from build123d import *

# Parameters (mm, degrees)
F0_R          = 10
F1_DEPTH      = 60
F1_DEPTH_BACK = 60
F2_R          = 2
F3_DEPTH      = 25
F5_START      = -10
F4_R          = 6
F5_DEPTH      = 15


with BuildPart() as f1:
    # F0 (on Top) → F1 (new body, two sides)
    with BuildSketch(Plane.XY) as f1_sk:
        with BuildLine():
            Line((-60, 10), (-60, 0))
            Line((-60, 0), (0, 0))
            Line((0, 0), (60, 0))
            Line((60, 0), (60, 10))
            Line((60, 10), (36.1375661614, 15.867864057))
            ThreePointArc((36.1375661614, 15.867864057), (25.2854930612, 21.0118409528), (17.3205080757, 30))
            ThreePointArc((17.3205080757, 30), (10, 37.3205080757), (0, 40))
            ThreePointArc((0, 40), (-10, 37.3205080757), (-17.3205080757, 30))
            ThreePointArc((-17.3205080757, 30), (-25.2854930612, 21.0118409528), (-36.1375661614, 15.867864057))
            Line((-36.1375661614, 15.867864057), (-60, 10))
        make_face()
        with Locations((0, 20)):
            Circle(F0_R, mode=Mode.SUBTRACT)
    extrude(amount=F1_DEPTH)
    extrude(f1_sk.sketch, amount=-F1_DEPTH_BACK)

    # F2 (on face) → F3 (cut)
    with BuildSketch(Plane.XZ):
        with Locations((-50, 50)):
            Circle(F2_R)
        with Locations((50, 50)):
            Circle(F2_R)
        with Locations((-50, -50)):
            Circle(F2_R)
        with Locations((50, -50)):
            Circle(F2_R)
    extrude(amount=-F3_DEPTH, mode=Mode.SUBTRACT)

    # F4 (on face) → F5 (cut)
    with BuildSketch(Plane.XZ.offset(F5_START)):
        with Locations((-50, 50)):
            Circle(F4_R)
        with Locations((50, -50)):
            Circle(F4_R)
        with Locations((-50, -50)):
            Circle(F4_R)
        with Locations((50, 50)):
            Circle(F4_R)
    extrude(amount=-F5_DEPTH, mode=Mode.SUBTRACT)


solid = f1.part
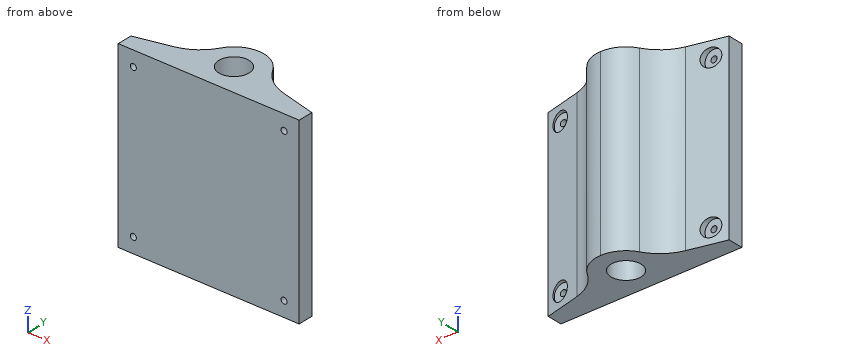
Geometry check sheet. Reference: the model listing, model coordinates, mm. Give positions to 0.01 mm unless a question says otherwise; leave off trailing zeros. Loops run counter-clockwise (first coordinate to the right, second up) from the corner with the lowest first, then second, coordinate; pieces in that order, holes last.
(1) Thickness scan on L1, parallel to Z at x = -50, y = 5.5; L2, parallel to Z at x = 45.5, y = 13.5; L3, parallel to X at y = 11.4, z = 50. Record the ranges inside material, lowest first.
From the geometry:
L1: z = -60 to -52, -48 to 48, 52 to 60
L2: z = -60 to -53.97, -46.03 to 46.03, 53.97 to 60
L3: x = -44 to -5.1, 5.1 to 44
(2) Section check A-A on z = 10. Record the cut outline in (x, y), then the cut area to 3 significant figures.
From the geometry:
outline: (-60, 0) - (60, 0) - (60, 10) - (36.14, 15.87) arc R30 cw to (17.32, 30) arc R20 ccw to (-17.32, 30) arc R30 cw to (-36.14, 15.87) - (-60, 10) - close; hole circle Ø20 at (0, 20)
area: 2,380 mm2
(3) Section check C-C on x = 6. Record the cut outline in (y, z), then the cut area to 3 significant figures.
From the geometry:
outline: (0, -60) - (12, -60) - (12, 60) - (0, 60) - close; (28, -60) - (39.08, -60) - (39.08, 60) - (28, 60) - close
area: 2,770 mm2
(4) Depth check by flat-ended pin: pin 1 Ø1.5 at (y, z) = (22, -0.5) entering from -X; pin 2 Ø8 at (x, z) = (-46, -26) entering from +Y; pin 3 Ø3.5 at (x, z) = (47.5, 49) entering from +Y; pin 4 Ø3 at (x, z) = (-50, 50) entering from -Y. Enter the tip coordinate at first touch or a pass-through.
From the geometry:
pin 1: stops at x = -24.97
pin 2: stops at y = 14.43
pin 3: stops at y = 10
pin 4: passes through
(5) Section check D-D on y = 20. Record the cut outline in (x, z).
From the geometry:
outline: (-26.72, -60) - (-10, -60) - (-10, 60) - (-26.72, 60) - close; (10, -60) - (26.72, -60) - (26.72, 60) - (10, 60) - close
(6) Section check B-B on z = 50. Record the cut outline in (x, y).
From the geometry:
outline: (-60, 0) - (-52, 0) - (-52, 10) - (-56, 10) - (-56, 10.98) - (-60, 10) - close; (-48, 0) - (48, 0) - (48, 10) - (44, 10) - (44, 13.93) - (36.14, 15.87) arc R30 cw to (17.32, 30) arc R20 ccw to (-17.32, 30) arc R30 cw to (-36.14, 15.87) - (-44, 13.93) - (-44, 10) - (-48, 10) - close; (52, 0) - (60, 0) - (60, 10) - (56, 10.98) - (56, 10) - (52, 10) - close; hole circle Ø20 at (0, 20)
